CAD build for the part. Positions are in the model's coordinates, mm. Face numbers are marked on the shaded views. Round coordinates to 2 decimals unless told otherwise and drop trailing zeros. Order: outer loops, then holes, each group sorted by start corner. A loop starts at its lowest first (then second) coordinate and runs counter-clockwise, first axis right, second up. Notation, with made-up numbers: M 46,-27 L 80,-27 A14 ccw 80,-3 Z; hole C 51.5,27.5 d7. An arc over 180 degrees is marked long. Put each result on its own line as item: value.
```python
from build123d import *

# Parameters (mm, degrees)
SKETCH1_R           = 36.2585
SKETCH1_R_2         = 3.175
BOSS_EXTRUDE1_DEPTH = 6.35
SKETCH2_W           = 6.604
SKETCH2_H           = 6.604
CUT_EXTRUDE1_DEPTH  = 10.16


with BuildPart() as part:
    # Sketch1 → Boss-Extrude1 (new body)
    with BuildSketch(Plane(origin=(0, 0, 0), x_dir=(1, 0, 0), z_dir=(0, 1, 0))):
        with Locations(Location((0, 0, 0), (0, 0, 270))):
            Circle(SKETCH1_R)
        with Locations(Location((0, 16.764, 0), (0, 0, 270))):
            Circle(SKETCH1_R_2, mode=Mode.SUBTRACT)
        with Locations(Location((0, -16.764, 0), (0, 0, 270))):
            Circle(SKETCH1_R_2, mode=Mode.SUBTRACT)
        with Locations(Location((-19.05, 0, 0), (0, 0, 270))):
            Circle(SKETCH1_R_2, mode=Mode.SUBTRACT)
        with Locations(Location((19.05, 0, 0), (0, 0, 270))):
            Circle(SKETCH1_R_2, mode=Mode.SUBTRACT)
    extrude(amount=BOSS_EXTRUDE1_DEPTH)

    # Sketch2 → Cut-Extrude1 (cut)
    with BuildSketch(Plane(origin=(0, 6.35, 0), x_dir=(1, 0, 0), z_dir=(0, 1, 0))):
        with Locations((-12.7635, 9.652)):
            Rectangle(SKETCH2_W, SKETCH2_H)
        with Locations((-12.7635, -9.652)):
            Rectangle(SKETCH2_W, SKETCH2_H)
        with Locations((12.7635, 9.652)):
            Rectangle(SKETCH2_W, SKETCH2_H)
        with Locations((12.7635, -9.652)):
            Rectangle(SKETCH2_W, SKETCH2_H)
    extrude(amount=-CUT_EXTRUDE1_DEPTH, mode=Mode.SUBTRACT)


solid = part.part
```
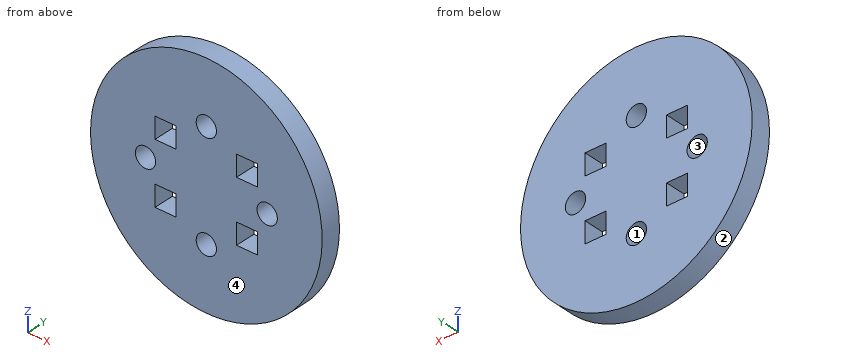
Item 1: Band-saw the part on C-C on z = -18. Give the cut face in (x, y), and give its area (3 significant figures).
Answers below:
outline: M -31.48,0 L -2.92,0 L -2.92,6.35 L -31.48,6.35 Z; M 2.92,0 L 31.48,0 L 31.48,6.35 L 2.92,6.35 Z
area: 363 mm²
Item 2: Band-saw the part on A-A on y = 3.75. State how many separate pieces and enclosed holes the cut face has, and give its area (3 significant figures).
Answers below:
separate pieces: 1
enclosed holes: 8
area: 3,830 mm²
Item 3: Probe line 1 along X through (y, z) = (1.75, 0) (1 decimal); line 2 along X through (y, z) = (2.5, -2); line 3 along Z through (x, y) = (11.5, 5.5). List the from-to ranges inside material, lowest first. Write a range as [from, to].
Answers below:
line 1: [-36.3, -22.2], [-15.9, 15.9], [22.2, 36.3]
line 2: [-36.2, -21.52], [-16.58, 16.58], [21.52, 36.2]
line 3: [-34.39, -12.95], [-6.35, 6.35], [12.95, 34.39]
Item 4: Pin check, flat tips, straight feed: P1, Ø1.9, axis at y = 2.5, z = -10.5, coming from the +X side; P2, Ø1.9, axis at x = 12, y = 3, coming from the +Z side; P3, Ø3, axis at x = 14, y = 4, coming from the -Z side. Stop position of each tip, or through.
Answers below:
P1: x = 34.98
P2: z = 34.53
P3: z = -34.04
Item 5: Mould opens along X. For the marked faces 1, 2, 3 and 4 say: pulls with the +X half, pulls with the -X half, needs draft (parallel to the pull), parting line crosses it, or undercut.
Answers below:
face 1: undercut
face 2: parting line crosses it
face 3: undercut
face 4: needs draft
Item 6: Band-saw the part on D-D on x = 21. Give the cut face in (y, z), and give its area (3 significant figures).
Answers below:
outline: M 0,-29.56 L 6.35,-29.56 L 6.35,-2.51 L 0,-2.51 Z; M 0,2.51 L 6.35,2.51 L 6.35,29.56 L 0,29.56 Z
area: 344 mm²
